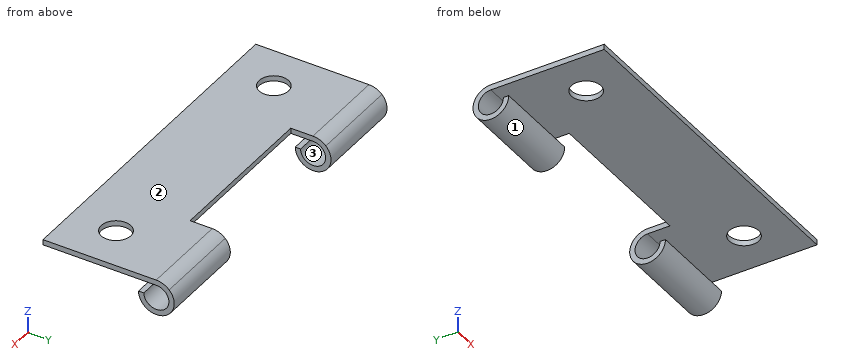
from build123d import *

# Parameters (mm, degrees)
SKETCH1_W           = 38.19
SKETCH1_H           = 10.19
BOSS_EXTRUDE1_DEPTH = 0.6
SKETCH2_W           = 10.06
SKETCH2_H           = 0.6
BOSS_EXTRUDE2_DEPTH = 4.5
BOSS_EXTRUDE3_DEPTH = 10.06
BOSS_EXTRUDE4_START = -10.06
BOSS_EXTRUDE4_DEPTH = 10.06
CUT_EXTRUDE1_DEPTH  = 40.672058177
SKETCH7_R           = 1.65
CUT_EXTRUDE2_DEPTH  = 10.01


with BuildPart() as part:
    # Sketch1 → Boss-Extrude1 (new body)
    with BuildSketch(Plane.XY):
        with Locations((19.095, -5.095)):
            Rectangle(SKETCH1_W, SKETCH1_H)
    extrude(amount=BOSS_EXTRUDE1_DEPTH)

    # Sketch2 → Boss-Extrude2 (add)
    with BuildSketch(Plane(origin=(0, 0, 0), x_dir=(1, 0, 0), z_dir=(0, 1, 0))):
        with Locations((5.03, -0.3)):
            Rectangle(SKETCH2_W, SKETCH2_H)
        with Locations((33.16, -0.3)):
            Rectangle(SKETCH2_W, SKETCH2_H)
    extrude(amount=BOSS_EXTRUDE2_DEPTH)

    # Sketch4 → Boss-Extrude3 (add)
    with BuildSketch(Plane(origin=(38.19, 0, 0), x_dir=(0, 0, -1), z_dir=(1, 0, 0))):
        with BuildLine():
            Line((0, 2.5), (-0.6, 2.5))
            ThreePointArc((-0.6, 2.5), (2.814213562, 3.914213562), (1.4, 0.5))
            Line((1.4, 0.5), (1.4, 1.1))
            ThreePointArc((1.4, 1.1), (2.389949494, 3.489949494), (0, 2.5))
        make_face()
    extrude(amount=-BOSS_EXTRUDE3_DEPTH)

    # Sketch5 → Boss-Extrude4 (add)
    with BuildSketch(Plane.ZY.offset(BOSS_EXTRUDE4_START)):
        with BuildLine():
            ThreePointArc((-1.4, 1.1), (-2.389949494, 3.489949494), (0, 2.5))
            Line((0, 2.5), (0, 3.928285686))
            ThreePointArc((0, 3.928285686), (-3.251563039, 3.256117924), (-1.4, 0.5))
            Line((-1.4, 0.5), (-1.4, 1.1))
        make_face()
        with BuildLine():
            Line((0, 3.928285686), (0, 2.5))
            Line((0, 2.5), (0.6, 2.5))
            ThreePointArc((0.6, 2.5), (0.443908891, 3.274596669), (0, 3.928285686))
        make_face()
    extrude(amount=BOSS_EXTRUDE4_DEPTH)

    # Sketch6 → Cut-Extrude1 (cut, through all)
    with BuildSketch(Plane.ZY):
        with BuildLine():
            Line((0, 3.928285686), (0, 4.5))
            Line((0, 4.5), (0.6, 4.5))
            Line((0.6, 4.5), (0.6, 2.47666439))
            ThreePointArc((0.6, 2.47666439), (0.44408843, 3.262031245), (0, 3.928285686))
        make_face()
    extrude(amount=-CUT_EXTRUDE1_DEPTH, mode=Mode.SUBTRACT)

    # Sketch7 → Cut-Extrude2 (cut)
    with BuildSketch(Plane(origin=(0, 0, 0), x_dir=(-1, 0, 0), z_dir=(0, 0, -1))):
        with Locations((-33.26, -5.095)):
            Circle(SKETCH7_R)
        with Locations((-4.93, -5.095)):
            Circle(SKETCH7_R)
    extrude(amount=-CUT_EXTRUDE2_DEPTH, mode=Mode.SUBTRACT)


solid = part.part
Could you check a few things on this model? Use its own coordinates, in mm. Face numbers are marked on the shaded views. Coordinates: 2 decimals unless noted, no trailing zeros. Order: outer loops, then holes, each group sorted by start corner. A loop starts at its lowest first (then second) coordinate and runs counter-clockwise, first axis right, second up.
Q1. Suppose I cut it at D-D on y = -1.5. Please give me the cut outline in (x, z).
Q2. Suppose I cut it at B-B on z = -0.7. Please give me the cut outline in (x, y).
Q3. Please list where these lines run through material, in increasing order: L1, parallel to Z at x = 31, y = 2.5; L2, parallel to Y at x = 6.5, z = -1.45; L3, parallel to Y at x = 25.5, z = 0.2.
Q4. Will these pins go through, and if not, where does the flat tip stop? pin 1 (0.5 mm diameter, centred on x = 17.5, z = 0.5, fed in from +Y); pin 2 (5.5 mm diameter, centred on x = 4.93, y = -5.095, fed in from -Z).
Q5. Thinking about a two-plate mould opening in Y: for the marked faces 1, 2 and 3, which applies, released by +Y, released by -Y, zero draft, split by the parting line, or undercut?
Q6. Suppose I cut it at A-A on x = 33.26. Please give me the cut outline in (y, z) (3 decimals).
Q7. Suppose I cut it at C-C on y = 3. Please give me the cut outline in (x, z).
Answer:
1. outline: (0, 0) - (38.19, 0) - (38.19, 0.6) - (0, 0.6) - close
2. outline: (0, 3.71) - (10.06, 3.71) - (10.06, 4.37) - (0, 4.37) - close; (28.13, 3.71) - (38.19, 3.71) - (38.19, 4.37) - (28.13, 4.37) - close
3. L1: z = -3.4 to -2.8, 0 to 0.6
3. L2: y = 0.5 to 1.1, 3.9 to 4.5
3. L3: y = -10.19 to 0
4. pin 1: stops at y = 0
4. pin 2: stops at z = 0
5. face 1: split by the parting line
5. face 2: zero draft
5. face 3: undercut
6. outline: (-10.19, 0) - (-6.745, 0) - (-6.745, 0.6) - (-10.19, 0.6) - close; (-3.445, 0) - (2.5, 0) arc R1.4 cw (long way) to (1.1, -1.4) - (0.5, -1.4) arc R2 ccw (long way) to (3.928, 0) arc R2.056 ccw to (2.477, 0.6) - (-3.445, 0.6) - close
7. outline: (0, -3.34) - (10.06, -3.34) - (10.06, -2.71) - (0, -2.71) - close; (0, -0.09) - (10.06, -0.09) - (10.06, 0.53) - (0, 0.53) - close; (28.13, -3.34) - (38.19, -3.34) - (38.19, -2.71) - (28.13, -2.71) - close; (28.13, -0.09) - (38.19, -0.09) - (38.19, 0.53) - (28.13, 0.53) - close
